```python
from build123d import *

# Parameters (mm, degrees)
F1_DEPTH = 3
F2_W     = 1
F2_H     = 20
F3_DEPTH = 12.5
F5_DEPTH = 10
F6_DEPTH = 10
F8_DEPTH = 3.1
F9_R     = 0.4162523321


with BuildPart() as f1:
    # F0 (on Front) → F1 (new body)
    with BuildSketch(Plane.XZ):
        Polygon((0, 54.4300840236), (-75, 24.4300840236), (-75, 4.4300840236), (0, 4.4300840236), align=None)
        Polygon((75, 24.4300840236), (0, 54.4300840236), (0, 4.4300840236), (75, 4.4300840236), align=None)
    extrude(amount=F1_DEPTH)

    # F2 (on face) → F3 (join)
    with BuildSketch(Plane.XZ.offset(3)):
        with Locations((-74.5, 14.4300840236)):
            Rectangle(F2_W, F2_H)
        with Locations((74.5, 14.4300840236)):
            Rectangle(F2_W, F2_H)
    extrude(amount=F3_DEPTH)

    # F4 (on face) → F5 (join)
    with BuildSketch(Plane(origin=(0, 0, 0), x_dir=(-1, 0, 0), z_dir=(0, 1, 0))):
        Polygon((-5, 4.4300840236), (0, 4.4300840236), (5, 4.4300840236), (5, 52.4300840236), (0, 52.4300840236), (-5, 52.4300840236), align=None)
    extrude(amount=F5_DEPTH)

    # F4 (on face) → F6 (join)
    with BuildSketch(Plane(origin=(0, 0, 0), x_dir=(-1, 0, 0), z_dir=(0, 1, 0))):
        Polygon((-5, 4.4300840236), (0, 4.4300840236), (5, 4.4300840236), (5, 52.4300840236), (0, 52.4300840236), (-5, 52.4300840236), align=None)
        Polygon((0, -45.5699159764), (0, 4.4300840236), (-5, 4.4300840236), align=None)
        Polygon((5, 4.4300840236), (0, 4.4300840236), (0, -45.5699159764), align=None)
        Polygon((0, 52.4300840236), (5, 52.4300840236), (0, 72.4300840236), align=None)
        Polygon((0, 72.4300840236), (-5, 52.4300840236), (0, 52.4300840236), align=None)
    extrude(amount=F6_DEPTH)

    # F7 (on face) → F8 (join)
    with BuildSketch(Plane.XZ):
        Polygon((-12.5, -39.854593575), (-0.5715322401, -39.854593575), (-1.5591000635, -29.9789153418), (-12.5, -34.854593575), align=None)
        Polygon((1.5591000635, -29.9789153418), (0.5715322401, -39.854593575), (12.5, -39.854593575), (12.5, -34.854593575), align=None)
    extrude(amount=-F8_DEPTH)

    # F9
    f9_edges = [f1.edges().sort_by_distance(p)[0] for p in [
        (0, 5, 72.430084),
    ]]
    fillet(f9_edges, radius=F9_R)


solid = f1.part
```
Geometry: final body of the model. Coordinates: model frame, mm. A direction names the side the tool comes from. Round coordinates to 2 decimals unless told otherwise and drop trailing zeros. Loops run counter-clockwise (first coordinate to the right, second up) from the corner with the lowest first, then second, coordinate; pieces in that order, holes last. Notation, with made-up numbers: (74.5, -21.75) -> (111.5, -21.75) arc R18 ccw to (111.5, -7.75) -> close; hole circle Ø9 at (76, 74). An arc over 180 degrees is marked (long way). Write each question's results on one line, items separated by ' | '.
Item 1: Cut plane D-D on z = 61. Return the cut outline in (x, y).
Answers below:
outline: (-2.86, 0) -> (2.86, 0) -> (2.86, 10) -> (-2.86, 10) -> close
Item 2: Set-up query: faces 1 (the face through (-2.734, 4.93, 61.494)), 2 (the face through (7.106, 1.528, -32.451)), 3 (the face through (32, 0, 23)), 4 (the face through (-33, 0, 23)), 5 (the face through (-7, 3.1, -36)). Return all of +Z, -Z, +X, -X, +Y, -Y with unobstructed straight access to the full face (end or side cutting, diameter ignored); none if empty.
Answers below:
face 1: +Z, -X, +Y, -Y | face 2: +X, +Y, -Y | face 3: +Z, +X, +Y | face 4: +Z, -X, +Y | face 5: -Z, -X, +Y
Item 3: Line query: probe 1 along X at (y, z) = (3, 13); probe 2 along Y at (x, z) = (26.5, 40.5); probe 3 along X at (y, z) = (7.75, -18.5). Output: solid intervals per line, ascending. Write a range as [from, to].
Answers below:
probe 1: x = [-5, 5] | probe 2: y = [-3, 0] | probe 3: x = [-2.71, 2.71]
Item 4: Cut plane A-A on y = -13.25. Return the cut outline in (x, z), and give its area (3 significant figures).
Answers below:
outline: (-75, 4.43) -> (-74, 4.43) -> (-74, 24.43) -> (-75, 24.43) -> close; (74, 4.43) -> (75, 4.43) -> (75, 24.43) -> (74, 24.43) -> close | area: 40.0 mm²
Item 5: Pin query (flat end, axial travel): pin 1 Ø20 at (x, z) = (4, -9.5) entering from -Y; pin 2 Ø25 at (x, z) = (-3.5, 18.5) entering from -Y; pin 3 Ø0.9 at (x, y) = (-5, 1) entering from -Z. Return the tip coordinate at first contact, or that it passes through.
Answers below:
pin 1: stops at y = 0 | pin 2: stops at y = -3 | pin 3: stops at z = -39.85
Item 6: Pull-direction query (X, two-part tool) for faces 6 (the face through (74, -9, 14)), 7 (the face through (-7, 2, -39.855)), 8 (the face through (-12.5, 2, -37)), 9 (the face through (-74, -9, 14)); classes: pulls with the +X half, pulls with the -X half, needs draft (parallel to the pull), parting line crosses it, or undercut.
Answers below:
face 6: undercut | face 7: needs draft | face 8: pulls with the -X half | face 9: undercut
Item 7: Cut plane B-B on z = 38. Return the cut outline in (x, y).
Answers below:
outline: (-41.08, -3) -> (41.08, -3) -> (41.08, 0) -> (5, 0) -> (5, 10) -> (-5, 10) -> (-5, 0) -> (-41.08, 0) -> close
Item 8: Cut plane C-C on x = 61. Return the cut outline in (y, z).
Answers below:
outline: (-3, 4.43) -> (0, 4.43) -> (0, 30.03) -> (-3, 30.03) -> close
